Geometry check sheet. Reference: the model listing, model coordinates, mm. Face numbers are marked on the shaded views. A direction names the side the tool comes from. Round coordinates to 2 decimals unless told otherwise and drop trailing zeros. Write each loop counter-clockwise with the first axis right and the second up, starting at its lowest first coordinate (ties: lowest second). Pieces come first, ordered by that corner, then holes. Notation, with made-up numbers: M 1.5,67 L 35.5,67 A36 ccw 35.5,101 Z; hole C 23.25,24.25 d5. An arc over 180 degrees is marked long. Use a Markdown table: item, result.
```python
from build123d import *

# Parameters (mm, degrees)
SKETCH1_W           = 23.862
SKETCH1_H           = 25
SKETCH1_R           = 1.1
BOSS_EXTRUDE1_DEPTH = 1.3
SKETCH2_W           = 8
SKETCH2_H           = 8
BOSS_EXTRUDE2_DEPTH = 2
SKETCH3_R           = 3.5
BOSS_EXTRUDE3_DEPTH = 2
FILLET1_R           = 2


with BuildPart() as part:
    # Sketch1 → Boss-Extrude1 (new body)
    with BuildSketch(Plane(origin=(0, 0, 0), x_dir=(1, 0, 0), z_dir=(0, 1, 0))):
        Rectangle(SKETCH1_W, SKETCH1_H)
        with Locations(Location((-9.931, -10.5, 0), (0, 0, 270))):
            Circle(SKETCH1_R, mode=Mode.SUBTRACT)
        with Locations(Location((2.569, -10.5, 0), (0, 0, 270))):
            Circle(SKETCH1_R, mode=Mode.SUBTRACT)
        with Locations(Location((-9.931, 10.5, 0), (0, 0, 270))):
            Circle(SKETCH1_R, mode=Mode.SUBTRACT)
        with Locations(Location((2.569, 10.5, 0), (0, 0, 270))):
            Circle(SKETCH1_R, mode=Mode.SUBTRACT)
    extrude(amount=BOSS_EXTRUDE1_DEPTH)

    # Sketch2 → Boss-Extrude2 (add)
    with BuildSketch(Plane.XZ):
        with Locations((2.469, 0)):
            Rectangle(SKETCH2_W, SKETCH2_H)
    extrude(amount=BOSS_EXTRUDE2_DEPTH)

    # Sketch3 → Boss-Extrude3 (add)
    with BuildSketch(Plane.XZ.offset(2)):
        with Locations(Location((2.469, 0, 0), (0, 0, 90))):
            Circle(SKETCH3_R)
    extrude(amount=BOSS_EXTRUDE3_DEPTH)

    # Fillet1
    fillet1_edges = [part.edges().sort_by_distance(p)[0] for p in [
        (11.931, 0.65, 12.5),
        (-11.931, 0.65, 12.5),
        (-11.931, 0.65, -12.5),
        (11.931, 0.65, -12.5),
    ]]
    fillet(fillet1_edges, radius=FILLET1_R)


solid = part.part
```
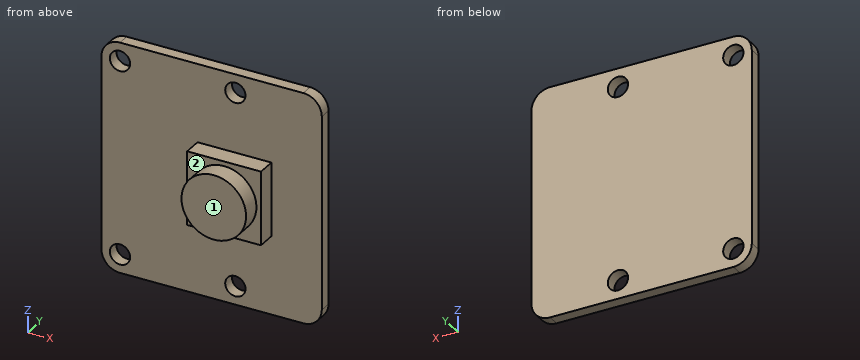
Item 1: Cross-section at B-B, the plane x = 0.5. Record the cut outline in (y, z).
Outcome:
| item | result |
|---|---|
| outline | M -4,-2.89 L -2,-2.89 L -2,-4 L 0,-4 L 0,-12.5 L 1.3,-12.5 L 1.3,12.5 L 0,12.5 L 0,4 L -2,4 L -2,2.89 L -4,2.89 Z |
Item 2: Material ranges on line 1 along X through (y, z) = (0.75, -10.5); line 2 along Y through (x, z) = (-0.25, -5.75); line 3 along X through (y, z) = (-1.75, 1), recorded low to high. Write a range as from..to.
Outcome:
| item | result |
|---|---|
| line 1 | x = -11.93..-11.03, -8.83..1.47, 3.67..11.93 |
| line 2 | y = 0..1.3 |
| line 3 | x = -1.53..6.47 |
Item 3: Access from +Z, -Z, +X, -X, +Y, -Y to the whole of each face (thin tool, end or side, straight path). Record for the marked faces 1 and 2.
Outcome:
| item | result |
|---|---|
| face 1 | +Z, -Z, +X, -X, -Y |
| face 2 | -Y |
Item 4: Cross-section at C-C, the plane y = -1.5. Record the cut outline in (x, z).
Outcome:
| item | result |
|---|---|
| outline | M -1.53,-4 L 6.47,-4 L 6.47,4 L -1.53,4 Z |
Item 5: Cross-section at A-A, the plane z = 0. Record the cut outline in (x, y).
Outcome:
| item | result |
|---|---|
| outline | M -11.93,0 L -1.53,0 L -1.53,-2 L -1.03,-2 L -1.03,-4 L 5.97,-4 L 5.97,-2 L 6.47,-2 L 6.47,0 L 11.93,0 L 11.93,1.3 L -11.93,1.3 Z |
Item 6: Go/stop test with flat-tipped pins: pin 1 (2 mm diameter, centred on x = -2.5, z = -6.5, fed in from -Y); pin 2 (1.8 mm diameter, centred on x = 2.569, z = 10.5, fed in from +Y); pin 3 (1 mm diameter, centred on x = 1.5, y = -1.5, fed in from -Z); pin 4 (1 mm diameter, centred on y = -1.5, z = 0.5, fed in from +X). Record where each tip stops, or that it passes through.
Outcome:
| item | result |
|---|---|
| pin 1 | stops at y = 0 |
| pin 2 | passes through |
| pin 3 | stops at z = -4 |
| pin 4 | stops at x = 6.47 |
Item 7: Cross-section at D-D, the plane z = 9. Record the cut outline in (x, y).
Outcome:
| item | result |
|---|---|
| outline | M -11.93,0 L 11.93,0 L 11.93,1.3 L -11.93,1.3 Z |
